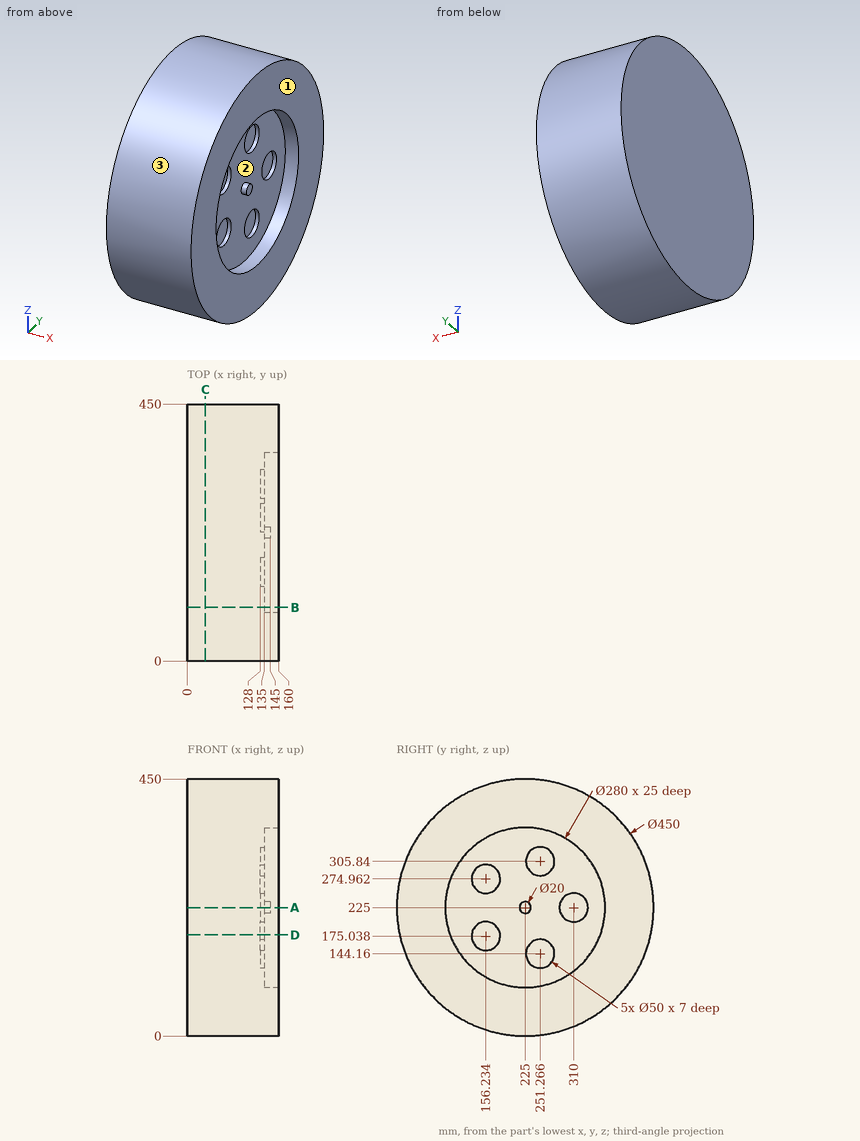
Could you check a few things on this drawing? It's one solid part, dimensions in mm from its lowest x, y, z. Coordinates: 2 decimals unless noted, no trailing zeros. Order: outer loops, then holes, each group sorted by start corner. A loop starts at its lowest first (then second) coordinate and runs counter-clockwise, first axis right, second up. Notation, with made-up numbers: M 67,68.5 L 77,68.5 A17 ccw 77,72.5 Z; hole C 85.25,42 d8. An arc over 180 degrees is marked long. Use one line per item in the form item = value. Start each with the question number.
1. Suppose I cut it at C-C on x = 31.5. Write out the boundary of the cut face in (y, z).
2. We'd pull the mould along Z, two halves only. Please class the marked faces 1, 2 and 3: +Z half, -Z half, draft (parallel to the pull), parting line (faces both ways), or undercut.
3. Suppose I cut it at B-B on y = 94. Write out the boundary of the cut face in (x, z).
4. Suppose I cut it at A-A on z = 225. Write out the boundary of the cut face in (x, y), then the cut area to 4 significant figures.
5. For pin 1 (1.5 mm diameter, centred on x = 70, z = 138.5, fed in from +Y); pin 2 (22 mm diameter, centred on y = 226, z = 229, fed in from +X); pin 3 (4 mm diameter, centred on x = 80.5, z = 315.5, fed in from +Y) (1 decimal); pin 4 (10 mm diameter, centred on y = 386, z = 323.5, fed in from -X), each with a flat end and sliding along its axis, tell me the tip position at first contact or that it passes through.
6. Please list where these lines run through material, in increasing order: line 1 (Z direction, x = 104, y = 221.5); line 2 (Z direction, x = 150, y = 175) (1 decimal); line 3 (Y direction, x = 114.5, z = 219).
7. Suppose I cut it at D-D on z = 177. Write out the boundary of the cut face in (x, y) (1 decimal).
Geometry says:
q1.outline = C 225,225 d450
q2.face_1 = draft
q2.face_2 = undercut
q2.face_3 = parting line
q3.outline = M 0,42.07 L 160,42.07 L 160,175.61 L 135,175.61 L 135,274.39 L 160,274.39 L 160,407.93 L 0,407.93 Z
q4.outline = M 0,0 L 160,0 L 160,85 L 135,85 L 135,215 L 145,215 L 145,235 L 135,235 L 135,285 L 128,285 L 128,335 L 135,335 L 135,365 L 160,365 L 160,450 L 0,450 Z
q4.area = 64,850 mm^2
q5.pin_1 = 433.02
q5.pin_2 = 145
q5.pin_3 = 431.9
q5.pin_4 = 0
q6.line_1 = 0.03 to 449.97
q6.line_2 = 5.6 to 94.2, 355.8 to 444.4
q6.line_3 = 0.08 to 449.92
q7.outline = M 0,5.2 L 160,5.2 L 160,93.5 L 135,93.5 L 135,131.3 L 128,131.3 L 128,181.2 L 135,181.2 L 135,356.5 L 160,356.5 L 160,444.8 L 0,444.8 Z
